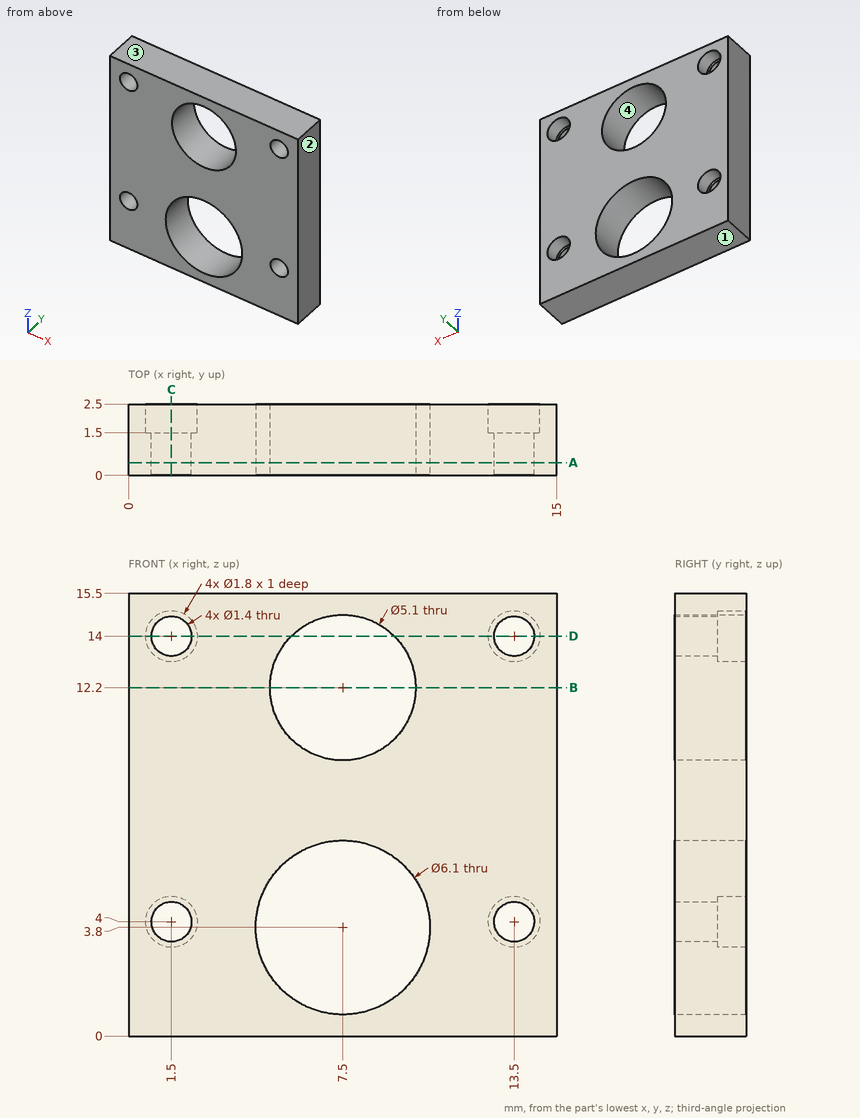
Verification items for this drawing (mm, ordinates from the low corner). Give positions to 0.01 mm unless a question says otherwise; leave off trailing zeros. Loops run counter-clockwise (first coordinate to the right, second up) from the corner with the lowest first, then second, coordinate; pieces in that order, holes last. Notation, with made-up numbers: (-14.75, 78) - (6.25, 78) arc R22 cw to (6.25, 86) - close; hole circle Ø4 at (61, 26.5). An arc over 180 degrees is marked (long way). Write item = value, one per line. Start each with the question number.
Q1. Thickness scan on line 1 (Z direction, x = 1.5, y = 0.4); line 2 (Z direction, x = 13.5, y = 2.1); line 3 (X direction, y = 1.4, z = 12.2). Record the ranges inside material, lowest first.
Q2. Mould release check, pull along Z, two halves, no side actions. Record for the marked faces 1, 2, 3 and 4: released by +Z, released by -Z, zero draft, split by the parting line, or undercut.
Q3. Cross-section at A-A, the plane y = 0.45. Enter the section's corners in (x, z), and give its area (3 significant figures).
Q4. Cross-section at D-D, the plane z = 14. Enter the section's corners in (x, y), and give its area (3 significant figures).
Q5. Depth check by flat-ended pin: P1, Ø1.8, axis at x = 13.5, z = 4, coming from the -Y side; P2, Ø1, axis at x = 9, z = 11, coming from the -Y side; P3, Ø1.6, axis at x = 1.5, z = 14, coming from the +Y side. Enter the tip coordinate at first touch or a pass-through.
Q6. Cross-section at C-C, the plane x = 1.5. Enter the section's corners in (y, z), and give its area (4 significant figures).
Q7. Cross-section at B-B, the plane z = 12.2. Enter the section's corners in (x, y), and give its area (4 significant figures).
Answer key:
q1.line_1 = 0 to 3.3, 4.7 to 13.3, 14.7 to 15.5
q1.line_2 = 0 to 3.1, 4.9 to 13.1, 14.9 to 15.5
q1.line_3 = 0 to 4.95, 10.05 to 15
q2.face_1 = released by -Z
q2.face_2 = zero draft
q2.face_3 = released by +Z
q2.face_4 = undercut
q3.outline = (0, 0) - (15, 0) - (15, 15.5) - (0, 15.5) - close; hole circle Ø1.4 at (1.5, 4); hole circle Ø1.4 at (1.5, 14); hole circle Ø6.1 at (7.5, 3.8); hole circle Ø5.1 at (7.5, 12.2); hole circle Ø1.4 at (13.5, 4); hole circle Ø1.4 at (13.5, 14)
q3.area = 177 mm^2
q4.outline = (0, 0) - (0.8, 0) - (0.8, 1.5) - (0.6, 1.5) - (0.6, 2.5) - (0, 2.5) - close; (2.2, 0) - (5.69, 0) - (5.69, 2.5) - (2.4, 2.5) - (2.4, 1.5) - (2.2, 1.5) - close; (9.31, 0) - (12.8, 0) - (12.8, 1.5) - (12.6, 1.5) - (12.6, 2.5) - (9.31, 2.5) - close; (14.2, 0) - (15, 0) - (15, 2.5) - (14.4, 2.5) - (14.4, 1.5) - (14.2, 1.5) - close
q4.area = 20.7 mm^2
q5.P1 = 0
q5.P2 = through
q5.P3 = 1.5
q6.outline = (0, 0) - (2.5, 0) - (2.5, 3.1) - (1.5, 3.1) - (1.5, 3.3) - (0, 3.3) - close; (0, 4.7) - (1.5, 4.7) - (1.5, 4.9) - (2.5, 4.9) - (2.5, 13.1) - (1.5, 13.1) - (1.5, 13.3) - (0, 13.3) - close; (0, 14.7) - (1.5, 14.7) - (1.5, 14.9) - (2.5, 14.9) - (2.5, 15.5) - (0, 15.5) - close
q6.area = 30.95 mm^2
q7.outline = (0, 0) - (4.95, 0) - (4.95, 2.5) - (0, 2.5) - close; (10.05, 0) - (15, 0) - (15, 2.5) - (10.05, 2.5) - close
q7.area = 24.75 mm^2
